Check sheet for the modelled part. Datum: model origin and axes. Units: mm. Round coordinates to 2 decimals unless told otherwise and drop trailing zeros. Loops run counter-clockwise (first coordinate to the right, second up) from the corner with the lowest first, then second, coordinate; pieces in that order, holes last. Notation, with made-up numbers: (67.5, 65.25) - (118.5, 65.25) arc R17 ccw to (118.5, 77.25) - close; hole circle Ø11 at (41, 58.25). An arc over 180 degrees is marked (long way). Return JSON: item names as keys, results as strings.
from build123d import *

# Parameters (mm, degrees)
SKETCH1_R             = 9.525
BOSS_EXTRUDE1_DEPTH   = 4.7625
F_6_CLEARANCE_HOLE1_D = 4.3053


with BuildPart() as part:
    # Sketch1 → Boss-Extrude1 (new body)
    with BuildSketch(Plane.XY):
        Polygon((-44.45, 10.16), (-85.56625, 44.958), (-97.63125, 44.958), (-97.63125, 0), (97.63125, 0), (97.63125, 44.958), (85.56625, 44.958), (44.45, 10.16), align=None)
        with Locations((-83.82, 21.59)):
            Circle(SKETCH1_R, mode=Mode.SUBTRACT)
        with Locations((83.82, 21.59)):
            Circle(SKETCH1_R, mode=Mode.SUBTRACT)
    extrude(amount=BOSS_EXTRUDE1_DEPTH)

    # #6 Clearance Hole1 (through all)
    with Locations(Plane.XY.offset(4.7625)):
        with Locations((89.408, 35.56), (58.42, 7.62), (-58.42, 7.62), (-89.408, 35.56)):
            Hole(F_6_CLEARANCE_HOLE1_D / 2)


solid = part.part
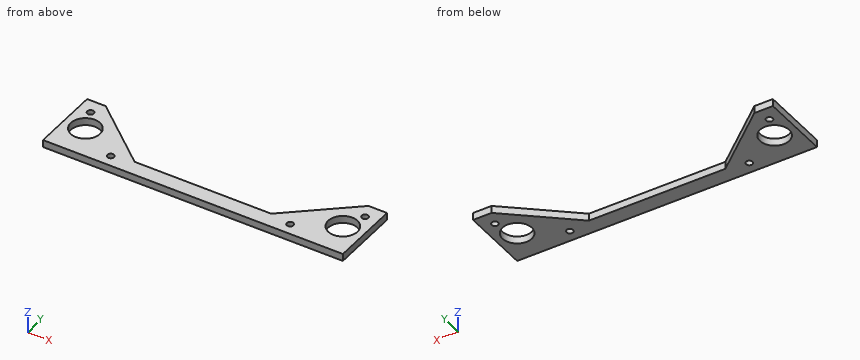
Q1. Scan lines: probe 1 along X at (y, z) = (37.5, 1.4); probe 2 along X at (y, z) = (25, 3.4); probe 3 along Y at (x, z) = (-42.5, 3). Record each from-to range of solid material in increasing order. Write a range as [from, to].
Answer key:
{"probe 1": "x = [-97.63, -90.34], [-88.48, -76.75], [76.75, 88.48], [90.34, 97.63]", "probe 2": "x = [-97.63, -92.71], [-74.93, -61.98], [61.98, 74.93], [92.71, 97.63]", "probe 3": "y = [0, 10.16]"}
Q2. Sectioned sample at A-A (x = 83.82). Enter the section's corners in (y, z) (1 decimal).
Answer key:
{"outline": "(0, 0) - (12.1, 0) - (12.1, 4.8) - (0, 4.8) - close; (31.1, 0) - (43.5, 0) - (43.5, 4.8) - (31.1, 4.8) - close"}
Q3. Sectioned sample at B-B (y = 21.59). Enter the section's corners in (x, z) (1 decimal), plus the area to 3 significant figures.
Answer key:
{"outline": "(-97.6, 0) - (-93.3, 0) - (-93.3, 4.8) - (-97.6, 4.8) - close; (-74.3, 0) - (-58, 0) - (-58, 4.8) - (-74.3, 4.8) - close; (58, 0) - (74.3, 0) - (74.3, 4.8) - (58, 4.8) - close; (93.3, 0) - (97.6, 0) - (97.6, 4.8) - (93.3, 4.8) - close", "area": "196 mm²"}
Q4. Sectioned sample at C-C (z = 3.6). Enter the section's corners in (x, y) (3 decimals), plus the area to 3 significant figures.
Answer key:
{"outline": "(-97.631, 0) - (97.631, 0) - (97.631, 44.958) - (85.566, 44.958) - (44.45, 10.16) - (-44.45, 10.16) - (-85.566, 44.958) - (-97.631, 44.958) - close; hole circle Ø19.05 at (-83.82, 21.59); hole circle Ø4.305 at (-89.408, 35.56); hole circle Ø4.305 at (-58.42, 7.62); hole circle Ø4.305 at (58.42, 7.62); hole circle Ø19.05 at (83.82, 21.59); hole circle Ø4.305 at (89.408, 35.56)", "area": "3,630 mm²"}
Q5. Depth check by flat-ended pin: P1, Ø1, axis at x = 18, z = 3.5, coming from the +Y side; P2, Ø1, axis at x = 61, z = 3, coming from the +Y side; P3, Ø3.5, axis at x = 58.42, y = 7.62, coming from the +Z side. Enter the tip coordinate at first touch or a pass-through.
Answer key:
{"P1": "stops at y = 10.16", "P2": "stops at y = 24.59", "P3": "passes through"}
Q6. Sectioned sample at D-D (x = -58.42). Enter the section's corners in (y, z), plus the area to 3 significant figures.
Answer key:
{"outline": "(0, 0) - (5.47, 0) - (5.47, 4.76) - (0, 4.76) - close; (9.77, 0) - (21.98, 0) - (21.98, 4.76) - (9.77, 4.76) - close", "area": "84.2 mm²"}
